Job drawing, mm, ordinate dimensions from the low corner. One solid piece. Round coordinates to 2 decimals unless told otherwise and drop trailing zeros. Order: outer loops, then holes, each group sorted by start corner. A loop starts at its lowest first (then second) coordinate and runs counter-clockwise, first axis right, second up. Notation, with made-up numbers: (2.5, -25.75) -> (28.5, -25.75) arc R36 cw to (28.5, 12.25) -> close; hole circle Ø4 at (23, 13.25). An arc over 180 degrees is marked (long way). Return JSON: item names as keys, results as strings. Group by question number.
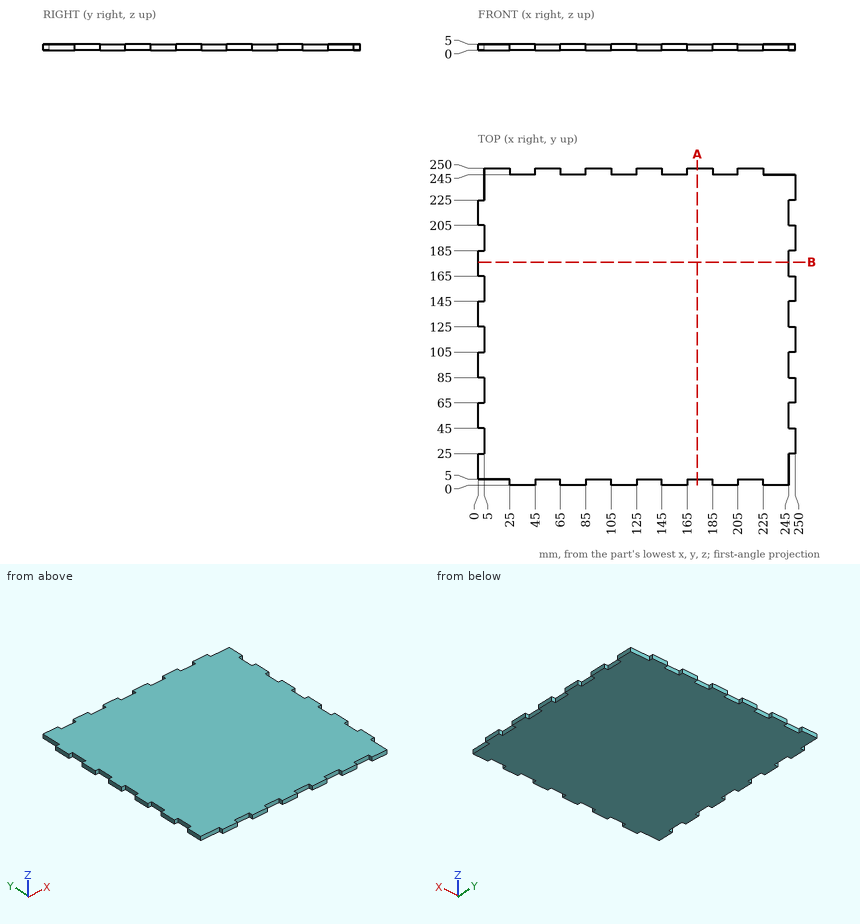
(1) Pin check, flat tips, straight feed: P1, Ø1.5, axis at x = 1.5, z = 2.5, coming from the +Y side; P2, Ø2.5, axis at y = 2.5, z = 2.5, coming from the -X side; P3, Ø1, axis at x = 161.5, z = 2.5, coming from the +Y side. Stop position of each tip, or through.
(2) Probe L1, parallel to X at y = 217, z = 4.85; L2, parallel to Y at x = 175, z = 0.45. List the from-to ranges inside material, lowest first. Write a range as [from, to].
(3) Saw through at B-B, the plane y = 176. List the corners of the cut face in (x, z).
(4) Saw through at A-A, the plane x = 173. List the corners of the cut face in (y, z), and give its area (4 significant figures).
Results are:
{
 "1": {"P1": "stops at y = 225", "P2": "stops at x = 25", "P3": "stops at y = 245"},
 "2": {"L1": "x = [0, 245]", "L2": "y = [5, 250]"},
 "3": {"outline": "(0, 0) -> (245, 0) -> (245, 5) -> (0, 5) -> close"},
 "4": {"outline": "(5, 0) -> (250, 0) -> (250, 5) -> (5, 5) -> close", "area": "1,225 mm^2"}
}
